```python
from build123d import *

# Parameters (mm, degrees)
SKETCH1_W           = 25.4
SKETCH1_H           = 50.8
SKETCH1_W_2         = 19.05
SKETCH1_H_2         = 44.45
BOSS_EXTRUDE1_DEPTH = 63.5
SKETCH2_R           = 3.3782
CUT_EXTRUDE3_DEPTH  = 73.955945611
SKETCH3_R           = 8.89
CUT_EXTRUDE4_DEPTH  = 73.955945611


with BuildPart() as part:
    # Sketch1 → Boss-Extrude1 (new, symmetric)
    with BuildSketch(Plane.XY):
        Rectangle(SKETCH1_W, SKETCH1_H)
        Rectangle(SKETCH1_W_2, SKETCH1_H_2, mode=Mode.SUBTRACT)
    extrude(amount=BOSS_EXTRUDE1_DEPTH, both=True)

    # Sketch2 → Cut-Extrude3 (cut, through all)
    with BuildSketch(Plane(origin=(12.7, 0, 0), x_dir=(0, 0, -1), z_dir=(1, 0, 0))):
        with Locations(Location((-22.225, 12.7, 0), (0, 0, 90))):
            Circle(SKETCH2_R)
        with Locations(Location((-22.225, -12.7, 0), (0, 0, 90))):
            Circle(SKETCH2_R)
        with Locations(Location((50.8, -12.7, 0), (0, 0, 90))):
            Circle(SKETCH2_R)
    extrude(amount=-CUT_EXTRUDE3_DEPTH, mode=Mode.SUBTRACT)

    # Sketch3 → Cut-Extrude4 (cut, through all)
    with BuildSketch(Plane(origin=(12.7, 0, 0), x_dir=(0, 0, -1), z_dir=(1, 0, 0))):
        with Locations(Location((48.26, 12.7, 0), (0, 0, 90))):
            Circle(SKETCH3_R)
    extrude(amount=-CUT_EXTRUDE4_DEPTH, mode=Mode.SUBTRACT)


solid = part.part
```
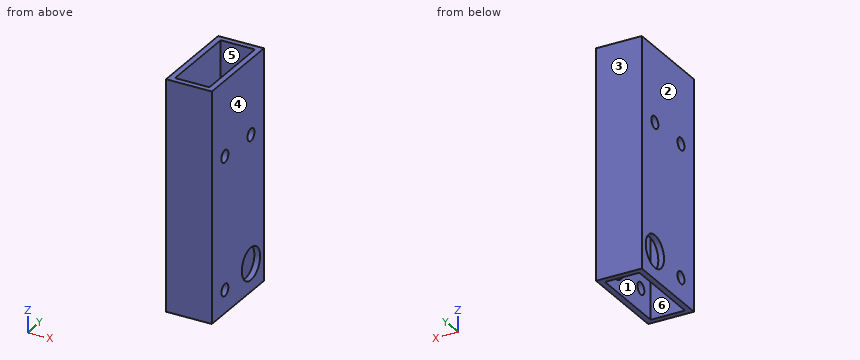
Geometry: final body of the model. Coordinates: model frame, mm. Face numbers are marked on the shaded views. A direction names the side the tool comes from. Round coordinates to 2 decimals unless told otherwise and drop trailing zeros. Write each loop counter-clockwise with the first axis right and the second up, starting at its lowest first coordinate (ties: lowest second). Pieces come first, ordered by that corner, then holes. Notation, with made-up numbers: M 61.5,-37.5 L 99.5,-37.5 A29 cw 99.5,-2.5 Z; hole C 70,-31.75 d3. An arc over 180 degrees is marked long. Answer in a Markdown table with one row per item. Add a question column.
(1) Cut plane D-D, the plane z = -50.8. Return the cut outline in (x, y) (3 decimals).
(2) Cut plane B-B, the plane x = 3.5. Return the cut outline in (y, z) (3 decimals).
(3) Cut plane C-C, the plane z = 39. Return the cut outline in (x, y) (3 decimals), then the cut area to 3 significant figures.
(4) Cut plane A-A, the plane y = 0. Return the cut outline in (x, z) (3 decimals).
(5) Ray query, L1, parallel to Z at x = 10.2, y = -12.7; L2, parallel to Z at x = -10.5, y = 12.7; L3, parallel to X at y = -8, z = 8 (3 decimals). Return the intervals inside material, ascending.
(6) Draft query along Y for the marked faces 3, 4, 5 and 6. Return one class per face: pulls with the +Y half, pulls with the -Y half, needs draft (parallel to the pull), parting line crosses it, or undercut.
(7) Reachability of the marked faces 1 and 2 from +Z, -Z, +X, -X, +Y, -Y: full face, straight path, thin tool, end or side. Return the list, or none.
Established:
| question | item | result |
|---|---|---|
| 1 | outline | M -12.7,-25.4 L 12.7,-25.4 L 12.7,-16.078 L 9.525,-16.078 L 9.525,-22.225 L -9.525,-22.225 L -9.525,-16.078 L -12.7,-16.078 Z; M -12.7,-9.322 L -9.525,-9.322 L -9.525,4.181 L -12.7,4.181 Z; M -12.7,21.219 L -9.525,21.219 L -9.525,22.225 L 9.525,22.225 L 9.525,21.219 L 12.7,21.219 L 12.7,25.4 L -12.7,25.4 Z; M 9.525,-9.322 L 12.7,-9.322 L 12.7,4.181 L 9.525,4.181 Z |
| 2 | outline | M -25.4,-63.5 L -22.225,-63.5 L -22.225,63.5 L -25.4,63.5 Z; M 22.225,-63.5 L 25.4,-63.5 L 25.4,63.5 L 22.225,63.5 Z |
| 3 | outline | M -12.7,-25.4 L 12.7,-25.4 L 12.7,25.4 L -12.7,25.4 Z; hole M -9.525,-22.225 L 9.525,-22.225 L 9.525,22.225 L -9.525,22.225 Z |
| 3 | area | 444 mm² |
| 4 | outline | M -12.7,-63.5 L -9.525,-63.5 L -9.525,63.5 L -12.7,63.5 Z; M 9.525,-63.5 L 12.7,-63.5 L 12.7,63.5 L 9.525,63.5 Z |
| 5 | L1 | -63.5 to -54.18, -47.42 to 18.85, 25.6 to 63.5 |
| 5 | L2 | -63.5 to -57.15, -39.37 to 18.85, 25.6 to 63.5 |
| 5 | L3 | -12.7 to -9.525, 9.525 to 12.7 |
| 6 | face 3 | pulls with the +Y half |
| 6 | face 4 | needs draft |
| 6 | face 5 | undercut |
| 6 | face 6 | undercut |
| 7 | face 1 | +Z, -Z |
| 7 | face 2 | +Z, -Z, -X, +Y, -Y |
